Geometry check sheet. Reference: the model listing, model coordinates, mm. A direction names the side the tool comes from. Give positions to 0.01 mm unless a question says otherwise; leave off trailing zeros. Write each loop counter-clockwise with the first axis right and the second up, starting at its lowest first coordinate (ties: lowest second). Pieces come first, ordered by that corner, then holes. Notation, with made-up numbers: (-22.5, -12) - (-0.5, -12) arc R12 ccw to (-0.5, 10) - close; hole circle Ø4 at (2.25, 81). An arc over 180 degrees is marked (long way). One line per question, with ' | ' between items. Start each with the question number.
Q1. Gauge pin test, flat ends, axial feed: P1, Ø4, axis at x = 12.37, y = 52.37, coming from the +Z side; P2, Ø12, axis at x = 4.5, y = 38, coming from the -Z side; P3, Ø10, axis at x = -41, z = -5, coming from the +Y side. Record the tip position at first contact, or that the pin passes through.
Q2. Section check A-A on y = 129. Record the boundary of the cut face in (x, z).
Q3. Section check C-C on x = 39. Record the boundary of the cut face in (y, z), and give its area (3 significant figures).
Q4. Section check D-D on y = 174.5. Record the boundary of the cut face in (x, z).
Q5. Release check for a two-part mould opening along Y. For faces 1 (the face through (-1, -2, 1)), 2 (the face through (0, 180, 32)), 3 (the face through (-3, 25, 30)) record: +Y half, -Y half, draft (parallel to the pull), parting line (faces both ways), or undercut.
Q6. Section check B-B on z = -33. Record the boundary of the cut face in (x, y), and give its area (3 significant figures).
Q7. Thickness scan on L1, parallel to Y at x = 2, z = -27; L2, parallel to Z at x = 17, y = 170.5; L3, parallel to X at y = 70, z = -3. Record the ranges inside material, lowest first. Write a range as [from, to].
Q8. Set-up check for faces 4 (the face through (0, 220, 0)), 5 (the face through (-11.056, 50.138, 26.041)), 6 (the face through (-59.94, -0.99, 2.64)), 7 (the face through (-2.6, 59.83, 30.99)), 8 (the face through (0, 40, 32)): record each of +Z, -Z, +X, -X, +Y, -Y from which the full face is reachable in a straight line by a thin tool's end or side.
```python
from build123d import *

# Parameters (mm, degrees)
SKETCH1_R           = 25
BOSS_EXTRUDE1_DEPTH = 220
SKETCH2_R           = 15
BOSS_EXTRUDE2_DEPTH = 30
SKETCH3_R           = 20
SKETCH3_R_2         = 1.5
BOSS_EXTRUDE4_DEPTH = 2
SKETCH4_R           = 60
BOSS_EXTRUDE5_DEPTH = 2


with BuildPart() as part:
    # Sketch1 → Boss-Extrude1 (new body)
    with BuildSketch(Plane(origin=(0, 0, 0), x_dir=(1, 0, 0), z_dir=(0, 1, 0))):
        Circle(SKETCH1_R)
    extrude(amount=BOSS_EXTRUDE1_DEPTH)

    # Sketch2 → Boss-Extrude2 (add)
    with BuildSketch(Plane.XY):
        with Locations((0, 180)):
            Circle(SKETCH2_R)
        with Locations((0, 40)):
            Circle(SKETCH2_R)
    extrude(amount=BOSS_EXTRUDE2_DEPTH)

    # Sketch3 → Boss-Extrude4 (add)
    with BuildSketch(Plane.XY.offset(30)):
        with Locations((0, 180)):
            Circle(SKETCH3_R)
        with Locations((0, 197.5)):
            Circle(SKETCH3_R_2, mode=Mode.SUBTRACT)
        with Locations((12.374368671, 192.374368671)):
            Circle(SKETCH3_R_2, mode=Mode.SUBTRACT)
        with Locations((17.5, 180)):
            Circle(SKETCH3_R_2, mode=Mode.SUBTRACT)
        with Locations((12.374368671, 167.625631329)):
            Circle(SKETCH3_R_2, mode=Mode.SUBTRACT)
        with Locations((0, 162.5)):
            Circle(SKETCH3_R_2, mode=Mode.SUBTRACT)
        with Locations((-12.374368671, 167.625631329)):
            Circle(SKETCH3_R_2, mode=Mode.SUBTRACT)
        with Locations((-17.5, 180)):
            Circle(SKETCH3_R_2, mode=Mode.SUBTRACT)
        with Locations((-12.374368671, 192.374368671)):
            Circle(SKETCH3_R_2, mode=Mode.SUBTRACT)
        with Locations((0, 40)):
            Circle(SKETCH3_R)
        with Locations((0, 57.5)):
            Circle(SKETCH3_R_2, mode=Mode.SUBTRACT)
        with Locations((12.374368671, 52.374368671)):
            Circle(SKETCH3_R_2, mode=Mode.SUBTRACT)
        with Locations((17.5, 40)):
            Circle(SKETCH3_R_2, mode=Mode.SUBTRACT)
        with Locations((12.374368671, 27.625631329)):
            Circle(SKETCH3_R_2, mode=Mode.SUBTRACT)
        with Locations((0, 22.5)):
            Circle(SKETCH3_R_2, mode=Mode.SUBTRACT)
        with Locations((-12.374368671, 27.625631329)):
            Circle(SKETCH3_R_2, mode=Mode.SUBTRACT)
        with Locations((-17.5, 40)):
            Circle(SKETCH3_R_2, mode=Mode.SUBTRACT)
        with Locations((-12.374368671, 52.374368671)):
            Circle(SKETCH3_R_2, mode=Mode.SUBTRACT)
    extrude(amount=BOSS_EXTRUDE4_DEPTH)

    # Sketch4 → Boss-Extrude5 (add)
    with BuildSketch(Plane.XZ):
        Circle(SKETCH4_R)
    extrude(amount=BOSS_EXTRUDE5_DEPTH)


solid = part.part
```
Working result:
1) P1: stops at z = 32 | P2: stops at z = -25 | P3: stops at y = 0
2) outline: circle Ø50 at (0, 0)
3) outline: (-2, -45.6) - (0, -45.6) - (0, 45.6) - (-2, 45.6) - close | area: 182 mm2
4) outline: (-19.23, 30) - (-13.96, 30) - (-13.96, 20.74) arc R25 ccw (long way) to (13.96, 20.74) - (13.96, 30) - (19.23, 30) - (19.23, 32) - (-19.23, 32) - close
5) face 1: -Y half | face 2: draft | face 3: undercut
6) outline: (-50.11, -2) - (50.11, -2) - (50.11, 0) - (-50.11, 0) - close | area: 200 mm2
7) L1: y = [-2, 0] | L2: z = [-18.33, 18.33], [30, 32] | L3: x = [-24.82, 24.82]
8) face 4: +Z, -Z, +X, -X, +Y | face 5: none | face 6: +Y, -Y | face 7: +Z | face 8: +Z, +X, -X, +Y
